Here's how the part is built. I have some questions about the finished solid (model axes, mm). Face numbers are marked on the shaded views. A direction names the side the tool comes from. Coordinates: 2 decimals unless noted, no trailing zeros. Write each loop counter-clockwise with the first axis right and the second up, starting at its lowest first coordinate (ties: lowest second). Pieces come first, ordered by that corner, then holes. Notation, with made-up numbers: M 80,72.25 L 122,72.25 A17 cw 122,102.25 Z; hole C 64,68 d1. An arc over 180 degrees is marked long. Write each question's results on one line, items separated by ' | '. Start each with the question number.
from build123d import *

# Parameters (mm, degrees)
SKETCH1_R           = 1.6
BOSS_EXTRUDE1_DEPTH = 1.2
SKETCH2_R           = 2.85
SKETCH2_W           = 2.937952631
SKETCH2_H           = 3.927283648
SKETCH2_W_2         = 4.2
SKETCH2_H_2         = 4.5
BOSS_EXTRUDE2_DEPTH = 1.2
SKETCH3_W           = 8
SKETCH3_H           = 8
BOSS_EXTRUDE3_DEPTH = 1.8
SKETCH4_R           = 4
BOSS_EXTRUDE4_DEPTH = 3.2
SKETCH5_R           = 0.6
CUT_EXTRUDE1_DEPTH  = 1
SKETCH7_W           = 7
SKETCH7_H           = 7
SKETCH7_W_2         = 3.728136851
SKETCH7_H_2         = 1.761566417
SKETCH7_H_3         = 1.704612402
SKETCH7_W_3         = 3.603269321
SKETCH7_H_4         = 1.768357774
SKETCH7_W_4         = 3.352143609
SKETCH7_H_5         = 1.732407439
SKETCH7_W_5         = 1.212415991
SKETCH7_H_6         = 2.614149225
SKETCH7_W_6         = 2.309899449
SKETCH7_H_7         = 0.895937988
SKETCH7_W_7         = 2.468868555
SKETCH7_H_8         = 1.120250043
SKETCH7_H_9         = 0.966414447
BOSS_EXTRUDE5_DEPTH = 1.2
SKETCH8_W           = 3
SKETCH8_H           = 8.5
BOSS_EXTRUDE6_DEPTH = 4
FILLET1_R           = 0.3
FILLET2_R           = 3
CHAMFER1_SIZE       = 2


with BuildPart() as part:
    # Sketch1 → Boss-Extrude1 (new body)
    with BuildSketch(Plane.XY):
        Polygon((0, 20), (-8.5, 20), (-8.5, 14), (0, 14), (0, 0), (36.5, 0), (36.5, 20), align=None)
        with Locations((-6, 17.5)):
            Circle(SKETCH1_R, mode=Mode.SUBTRACT)
        with Locations((34, 2.5)):
            Circle(SKETCH1_R, mode=Mode.SUBTRACT)
        with Locations((34, 17.5)):
            Circle(SKETCH1_R, mode=Mode.SUBTRACT)
    extrude(amount=BOSS_EXTRUDE1_DEPTH)

    # Sketch2 → Boss-Extrude2 (add)
    with BuildSketch(Plane.XY.offset(1.2)):
        with Locations((2.9, 5.049940133)):
            Circle(SKETCH2_R)
        with Locations((27.263972555, 5.991759132)):
            Rectangle(SKETCH2_W, SKETCH2_H)
        with Locations((-0.408107806, 17.235427956)):
            Rectangle(SKETCH2_W_2, SKETCH2_H_2)
    extrude(amount=BOSS_EXTRUDE2_DEPTH)

    # Sketch3 → Boss-Extrude3 (add)
    with BuildSketch(Plane.XY.offset(1.2)):
        with Locations((13, 10.3)):
            Rectangle(SKETCH3_W, SKETCH3_H)
    extrude(amount=BOSS_EXTRUDE3_DEPTH)

    # Sketch4 → Boss-Extrude4 (add)
    with BuildSketch(Plane.XY.offset(3)):
        with Locations((13, 10.3)):
            Circle(SKETCH4_R)
    extrude(amount=BOSS_EXTRUDE4_DEPTH)

    # Sketch5 → Cut-Extrude1 (cut)
    with BuildSketch(Plane.XY.offset(6.2)):
        with Locations((13, 10.3)):
            Circle(SKETCH5_R)
    extrude(amount=-CUT_EXTRUDE1_DEPTH, mode=Mode.SUBTRACT)

    # Sketch7 → Boss-Extrude5 (add)
    with BuildSketch(Plane(origin=(0, 0, 0), x_dir=(-1, 0, 0), z_dir=(0, 0, -1))):
        with Locations((-10.5, 11)):
            Rectangle(SKETCH7_W, SKETCH7_H)
        with Locations((-21.140690462, 1.973810546)):
            Rectangle(SKETCH7_W_2, SKETCH7_H_2)
        with Locations((-21.140690462, 4.459014526)):
            Rectangle(SKETCH7_W_2, SKETCH7_H_3)
        with Locations((-19.339055802, 16.82217617)):
            Rectangle(SKETCH7_W_3, SKETCH7_H_4)
        with Locations((-6.335774559, 4.965027996)):
            Rectangle(SKETCH7_W_4, SKETCH7_H_5)
        with Locations((0.606207996, 17.481290904)):
            Rectangle(SKETCH7_W_5, SKETCH7_H_6)
        with Locations((-18.692370866, 14.947968994)):
            Rectangle(SKETCH7_W_6, SKETCH7_H_7)
        with Locations((-25.431234808, 4.404902976)):
            Rectangle(SKETCH7_W_7, SKETCH7_H_8)
        with Locations((-25.431234808, 1.951905582)):
            Rectangle(SKETCH7_W_7, SKETCH7_H_9)
    extrude(amount=BOSS_EXTRUDE5_DEPTH)

    # Sketch8 → Boss-Extrude6 (add)
    with BuildSketch(Plane.XY.offset(1.2)):
        with Locations((20.7, 7.75)):
            Rectangle(SKETCH8_W, SKETCH8_H)
    extrude(amount=BOSS_EXTRUDE6_DEPTH)

    # Fillet1
    fillet1_edges = [part.edges().sort_by_distance(p)[0] for p in [
        (9, 10.3, 6.2),
    ]]
    fillet(fillet1_edges, radius=FILLET1_R)

    # Fillet2
    fillet2_edges = [part.edges().sort_by_distance(p)[0] for p in [
        (36.5, 20, 0.6),
        (36.5, 0, 0.6),
        (-8.5, 14, 0.6),
        (-8.5, 20, 0.6),
    ]]
    fillet(fillet2_edges, radius=FILLET2_R - 0.0001)  # a hair under: the kernel refuses the full size

    # Chamfer1
    chamfer1_edges = [part.edges().sort_by_distance(p)[0] for p in [
        (0, 0, 0.6),
    ]]
    chamfer(chamfer1_edges, length=CHAMFER1_SIZE)


solid = part.part
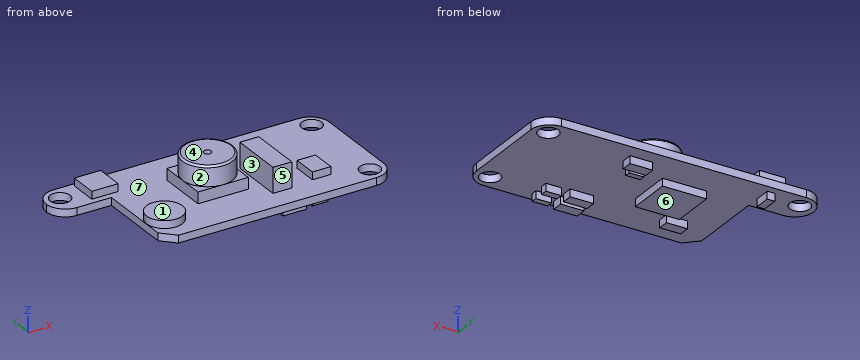
1) Please list where these lines run through material, in increasing order: line 1 (Y direction, x = 34, z = 0.5); line 2 (Z direction, x = 31, y = 5.25); line 3 (Y direction, x = 10.5, z = 1.75). Write a range as [from, to].
2) We'd pull the mould along X, two halves only. Please class the marked faces 6 and 7: pulls with the +X half, pulls with the -X half, needs draft (parallel to the pull), parting line crosses it, or undercut.
3) For the marked faces 1, 2, 3, 4 and 5, which set-ups out of +Z, -Z, +X, -X, +Y, -Y let a thin tool reach every point of the face, with its end or its side?
4) I want a section at A-A, the plane x = -6. Write out the boundary of the cut face in (y, z).
5) I want a section at C-C, the plane x = 34. Write out the boundary of the cut face in (y, z), then the cut area to 3 significant figures.
6) I want a section at D-D, the plane z = -0.5. Give the number of separate pieces and of enclosed holes in the cut face, then the cut area to 3 significant figures.
7) I want a section at B-B, the plane y = 18.25. Write out the boundary of the cut face in (x, z), then the cut area to 3 significant figures.
8) For pin 1 Ø1.5 at (x, y) = (20.5, 16.5) entering from +Z; pin 2 Ø0.6 at (x, z) = (7, -0.5) entering from +Y; pin 3 Ø1.5 at (x, y) = (21, 8) entering from +Z; pin 4 Ø2 at (y, z) = (12, 2) entering from +X, each with a flat end and sliding along its axis, tell me the tip position at first contact or that it passes through.
Output:
1) line 1: y = [0.04, 0.9], [4.1, 15.9], [19.1, 19.96] | line 2: z = [0, 1.2] | line 3: y = [6.3, 14.3]
2) face 6: needs draft | face 7: undercut
3) face 1: +Z, -X, +Y, -Y | face 2: +Z | face 3: +Z, +Y, -Y | face 4: +Z, +X, -X, +Y, -Y | face 5: +Z, +X, -Y
4) outline: M 14.04,0 L 15.9,0 L 15.9,1.2 L 14.04,1.2 Z; M 19.1,0 L 19.96,0 L 19.96,1.2 L 19.1,1.2 Z
5) outline: M 0.04,0 L 0.9,0 L 0.9,1.2 L 0.04,1.2 Z; M 4.1,0 L 15.9,0 L 15.9,1.2 L 4.1,1.2 Z; M 19.1,0 L 19.96,0 L 19.96,1.2 L 19.1,1.2 Z | area: 16.2 mm2
6) separate pieces: 9 | enclosed holes: 0 | area: 84.5 mm2
7) outline: M -8.23,0 L -7.41,0 L -7.41,1.2 L -8.23,1.2 Z; M -4.59,0 L -1.21,0 L -1.21,-1.2 L 0,-1.2 L 0,0 L 32.59,0 L 32.59,1.2 L 1.69,1.2 L 1.69,2.4 L -2.51,2.4 L -2.51,1.2 L -4.59,1.2 Z; M 35.41,0 L 36.23,0 L 36.23,1.2 L 35.41,1.2 Z | area: 53.1 mm2
8) pin 1: stops at z = 1.2 | pin 2: stops at y = 14.5 | pin 3: stops at z = 5.2 | pin 4: stops at x = 36.5
